from build123d import *

# Parameters (mm, degrees)
SKETCH_1_W          = 18
SKETCH_1_H          = 6
SKETCH_1_R          = 1.5
EXTRUDE_1_DEPTH     = 1.5
SKETCH_2_R          = 1.5
CUT_EXTRUDE_1_DEPTH = 10.949874371
FILLET_1_R          = 0.5


with BuildPart() as part:
    # 草图1 → 凸台-拉伸1 (new, symmetric)
    with BuildSketch(Plane.XY):
        Rectangle(SKETCH_1_W, SKETCH_1_H)
        Circle(SKETCH_1_R, mode=Mode.SUBTRACT)
    extrude(amount=EXTRUDE_1_DEPTH, both=True)

    # 草图2 → 切除-拉伸1 (cut, through all)
    with BuildSketch(Plane.XY.offset(1.5)):
        with Locations((-5.5, 0)):
            Circle(SKETCH_2_R)
        with Locations((5.5, 0)):
            Circle(SKETCH_2_R)
    extrude(amount=-CUT_EXTRUDE_1_DEPTH, mode=Mode.SUBTRACT)

    # 圆角1
    fillet_1_edges = [part.edges().sort_by_distance(p)[0] for p in [
        (-9, 3, 0),
        (9, 3, 0),
        (9, -3, 0),
        (-9, -3, 0),
    ]]
    fillet(fillet_1_edges, radius=FILLET_1_R)


solid = part.part
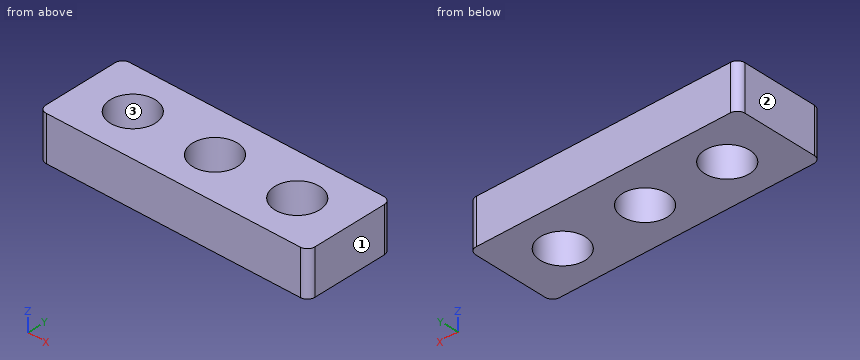
Verification items for the finished model (mm, model axes). Face numbers are marked on the shaded views. Coordinates: 2 decimals unless noted, no trailing zeros. Write each loop counter-clockwise with the first axis right and the second up, starting at its lowest first coordinate (ties: lowest second). Pieces come first, ordered by that corner, then holes. Notation, with made-up numbers: (-16.5, -31) -> (13.5, -31) arc R34 ccw to (13.5, 5) -> close; hole circle Ø5 at (-16.75, 18.25). An arc over 180 degrees is marked (long way). One line per item, written item: value. Start each with the question number.
Q1. Cross-section at C-C on z = -0.3. Enter the section's corners in (x, y).
Q2. Go/stop test with flat-tipped pins: P1, Ø1.8, axis at x = -5.5, y = 0, coming from the +Z side; P2, Ø3, axis at x = -5.5, y = -1, coming from the -Z side. Record where each tip stops, or that it passes through.
Q3. Thickness scan on L1, parallel to Y at x = 0, z = 0.5; L2, parallel to X at y = -1, z = -0.7; L3, parallel to X at y = 0.75, z = 0.6. Record the ranges inside material, lowest first. Write a range as from..to.
Q4. Cross-section at A-A on x = 5.5. Enter the section's corners in (y, z).
Q5. Cross-section at B-B on y = 0. Enter the section's corners in (x, z), and give its area (3 significant figures).
Q6. Cross-section at D-D on x = -6. Enter the section's corners in (y, z), and give its area (3 significant figures).
Q7. Mould release check, pull along X, two halves, no side actions. Record for the marked faces 1, 2 and 3: pulls with the +X half, pulls with the -X half, needs draft (parallel to the pull), parting line crosses it, or undercut.
Checked values:
1. outline: (-9, -2.5) arc R0.5 ccw to (-8.5, -3) -> (8.5, -3) arc R0.5 ccw to (9, -2.5) -> (9, 2.5) arc R0.5 ccw to (8.5, 3) -> (-8.5, 3) arc R0.5 ccw to (-9, 2.5) -> close; hole circle Ø3 at (-5.5, 0); hole circle Ø3 at (0, 0); hole circle Ø3 at (5.5, 0)
2. P1: passes through
2. P2: stops at z = -1.5
3. L1: y = -3..-1.5, 1.5..3
3. L2: x = -9..-6.62, -4.38..-1.12, 1.12..4.38, 6.62..9
3. L3: x = -9..-6.8, -4.2..-1.3, 1.3..4.2, 6.8..9
4. outline: (-3, -1.5) -> (-1.5, -1.5) -> (-1.5, 1.5) -> (-3, 1.5) -> close; (1.5, -1.5) -> (3, -1.5) -> (3, 1.5) -> (1.5, 1.5) -> close
5. outline: (-9, -1.5) -> (-7, -1.5) -> (-7, 1.5) -> (-9, 1.5) -> close; (-4, -1.5) -> (-1.5, -1.5) -> (-1.5, 1.5) -> (-4, 1.5) -> close; (1.5, -1.5) -> (4, -1.5) -> (4, 1.5) -> (1.5, 1.5) -> close; (7, -1.5) -> (9, -1.5) -> (9, 1.5) -> (7, 1.5) -> close
5. area: 27.0 mm²
6. outline: (-3, -1.5) -> (-1.41, -1.5) -> (-1.41, 1.5) -> (-3, 1.5) -> close; (1.41, -1.5) -> (3, -1.5) -> (3, 1.5) -> (1.41, 1.5) -> close
6. area: 9.51 mm²
7. face 1: pulls with the +X half
7. face 2: pulls with the -X half
7. face 3: undercut
